The drawing under review shows one solid part. Ordinate dimensions are in mm from its lowest x, y, z. A direction names the side the tool comes from. Coordinates: 2 decimals unless noted, no trailing zeros. Loops run counter-clockwise (first coordinate to the right, second up) from the corner with the lowest first, then second, coordinate; pieces in that order, holes last. Notation, with made-up numbers: M 45,84 L 50,84 A12 cw 50,88 Z; hole C 42.5,18 d5. An arc over 180 degrees is marked long. Answer as a JSON object with one key per item and string values. Group by question number.
1. Consider section C-C (y = 8.75). State the section outline as (x, z) points.
2. Consider section D-D (x = 2). State the section outline as (y, z) points.
3. To check wall thickness, follow probe 1 along X at (y, z) = (9.5, 0.35); probe 2 along Y at (x, z) = (1.75, 0.5). State the ranges of each line that lie inside material, in increasing order.
4. Machinability: for the marked faces 1, 2 and 3, which of the approach directions +Z, -Z, +X, -X, +Y, -Y give a long, thin tool a straight path to every point of the face, cutting with its end or side? Answer none if there is none.
5. Consider section A-A (z = 0.7). State the section outline as (x, y) points.
6. Consider section B-B (x = 4). State the section outline as (y, z) points, then the cut area to 3 significant figures.
7. Draft analysis for pull direction Y (two halves, no side actions). For the marked faces 4, 5 and 6, state which applies: +Y half, -Y half, draft (parallel to the pull), parting line (faces both ways), or undercut.
8. Insertion check: pin 1 (0.5 mm diameter, centred on y = 9.5, z = 0.5, fed in from -X). The pin has a flat end and moves straight along its axis. Give the tip position at first contact, or say it passes through.
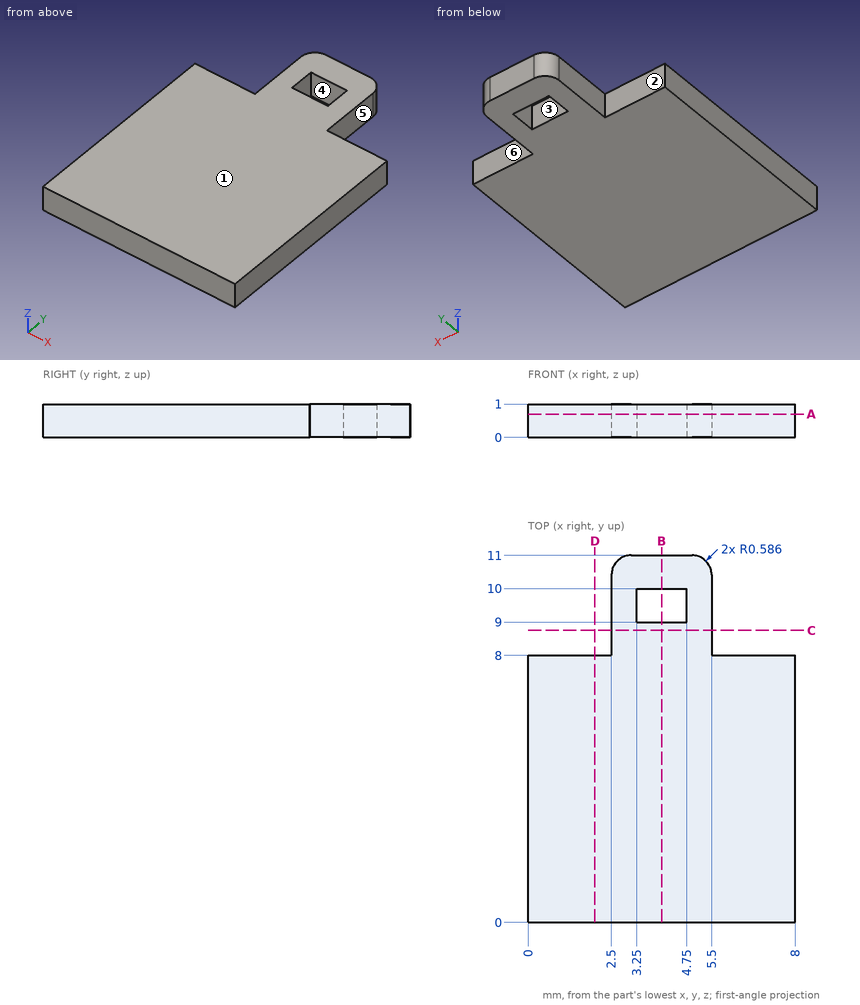
Findings below:
{
 "1": {"outline": "M 2.5,0 L 5.5,0 L 5.5,1 L 2.5,1 Z"},
 "2": {"outline": "M 0,0 L 8,0 L 8,1 L 0,1 Z"},
 "3": {"probe 1": "x = 2.5 to 3.25, 4.75 to 5.5", "probe 2": "y = 0 to 8"},
 "4": {"face 1": "+Z, +X, -X, +Y, -Y", "face 2": "+Z, -Z, -X, +Y", "face 3": "+Z, -Z"},
 "5": {"outline": "M 0,0 L 8,0 L 8,8 L 5.5,8 L 5.5,10.41 A0.59 ccw 4.91,11 L 3.09,11 A0.59 ccw 2.5,10.41 L 2.5,8 L 0,8 Z; hole M 3.25,9 L 4.75,9 L 4.75,10 L 3.25,10 Z"},
 "6": {"outline": "M 0,0 L 9,0 L 9,1 L 0,1 Z; M 10,0 L 11,0 L 11,1 L 10,1 Z", "area": "10.0 mm^2"},
 "7": {"face 4": "undercut", "face 5": "draft", "face 6": "+Y half"},
 "8": {"pin 1": "stops at x = 2.5"}
}
